from build123d import *

# Parameters (mm, degrees)
SKETCH1_R               = 3.175
SKETCH1_R_2             = 2.25
BOSS_EXTRUDE1_DEPTH     = 35
SKETCH2_W               = 13.029993618
SKETCH2_H               = 25
CUT_EXTRUDE1_DEPTH      = 2
CUT_EXTRUDE1_DEPTH_BACK = 5
SKETCH3_R               = 0.889
F_2_56_HOLE_DEPTH       = 3
SKETCH4_R               = 3.175
SKETCH4_R_2             = 2.25
BOSS_EXTRUDE2_DEPTH     = 120


with BuildPart() as part:
    # Sketch1 → Boss-Extrude1 (new body)
    with BuildSketch(Plane.XY):
        Circle(SKETCH1_R)
        Circle(SKETCH1_R_2, mode=Mode.SUBTRACT)
    extrude(amount=BOSS_EXTRUDE1_DEPTH)

    # Sketch2 → Cut-Extrude1 (cut, two sides)
    with BuildSketch(Plane(origin=(0, 0, 0), x_dir=(1, 0, 0), z_dir=(0, 1, 0))) as cut_extrude1_sk:
        with Locations((0.986854582, -17.5)):
            Rectangle(SKETCH2_W, SKETCH2_H)
    extrude(amount=CUT_EXTRUDE1_DEPTH, mode=Mode.SUBTRACT)
    extrude(cut_extrude1_sk.sketch, amount=-CUT_EXTRUDE1_DEPTH_BACK, mode=Mode.SUBTRACT)

    # Sketch3 → 2-56 hole (cut)
    with BuildSketch(Plane(origin=(0, 2, 0), x_dir=(-1, 0, 0), z_dir=(0, -1, 0))):
        with Locations((0, -20)):
            Circle(SKETCH3_R)
    extrude(amount=-F_2_56_HOLE_DEPTH, mode=Mode.SUBTRACT)

    # Sketch4 → Boss-Extrude2 (add)
    with BuildSketch(Plane.XY.offset(35)):
        Circle(SKETCH4_R)
        Circle(SKETCH4_R_2, mode=Mode.SUBTRACT)
    extrude(amount=BOSS_EXTRUDE2_DEPTH)


solid = part.part
The model under review builds one solid part; all positions refer to its coordinate system, in mm. Coordinates: 2 decimals unless noted, no trailing zeros. Write each loop counter-clockwise with the first axis right and the second up, starting at its lowest first coordinate (ties: lowest second). Pieces come first, ordered by that corner, then holes. Notation, with made-up numbers: (-8, 13) - (0, 13) arc R11 cw to (0, 27) - close; hole circle Ø4 at (1.5, 47). An arc over 180 degrees is marked (long way). Answer as a JSON object with one key per item and string values. Group by question number.
1. Clearance check with flat-ended pins moving along their axes: pin 1 Ø1 at (y, z) = (-0.5, 120.5) entering from +X (3 decimals); pin 2 Ø1.6 at (x, z) = (-1.5, 17) entering from -Y; pin 3 Ø1 at (y, z) = (1, 85.5) entering from -X. State where each tip first meets the part, or that it passes through.
2. Mouldability with a two-part tool opening along Z and no side actions: class faces 1 (the face through (1.4, -2.1, 155)), 2 (the face through (0, -3, 30)), 3 (the face through (-0.29, 2.23, 93.64)), 4 (the face through (0.7, -2.3, 5)) as pulls with the +Z half, pulls with the -Z half, needs draft (parallel to the pull), parting line crosses it, or undercut.
3. Add section A-A (y = 0). Give the boundary of the cut face in (x, z) (3 decimals), plus the area to 4 significant figures.
4. Add section B-B (z = 58). Give the boundary of the cut face in (x, y) (3 decimals), plus the area to 3 significant figures.
5. To check wall thickness, follow probe 1 along X at (y, z) = (0.25, 41); probe 2 along Z at (x, y) = (2.25, -2); probe 3 along Z at (x, y) = (0, 3). State the ranges of each line that lie inside material, in increasing order.
Findings:
{
 "1": {"pin 1": "x = 3.175", "pin 2": "y = 2", "pin 3": "x = -3.14"},
 "2": {"face 1": "pulls with the +Z half", "face 2": "undercut", "face 3": "needs draft", "face 4": "undercut"},
 "3": {"outline": "(-3.175, 0) - (-2.25, 0) - (-2.25, 5) - (-3.175, 5) - close; (-3.175, 30) - (-2.25, 30) - (-2.25, 155) - (-3.175, 155) - close; (2.25, 0) - (3.175, 0) - (3.175, 5) - (2.25, 5) - close; (2.25, 30) - (3.175, 30) - (3.175, 155) - (2.25, 155) - close", "area": "240.5 mm²"},
 "4": {"outline": "circle Ø6.35 at (0, 0); hole circle Ø4.5 at (0, 0)", "area": "15.8 mm²"},
 "5": {"probe 1": "-3.17 to -2.24, 2.24 to 3.17", "probe 2": "0 to 5, 30 to 155", "probe 3": "0 to 19.11, 20.89 to 155"}
}
